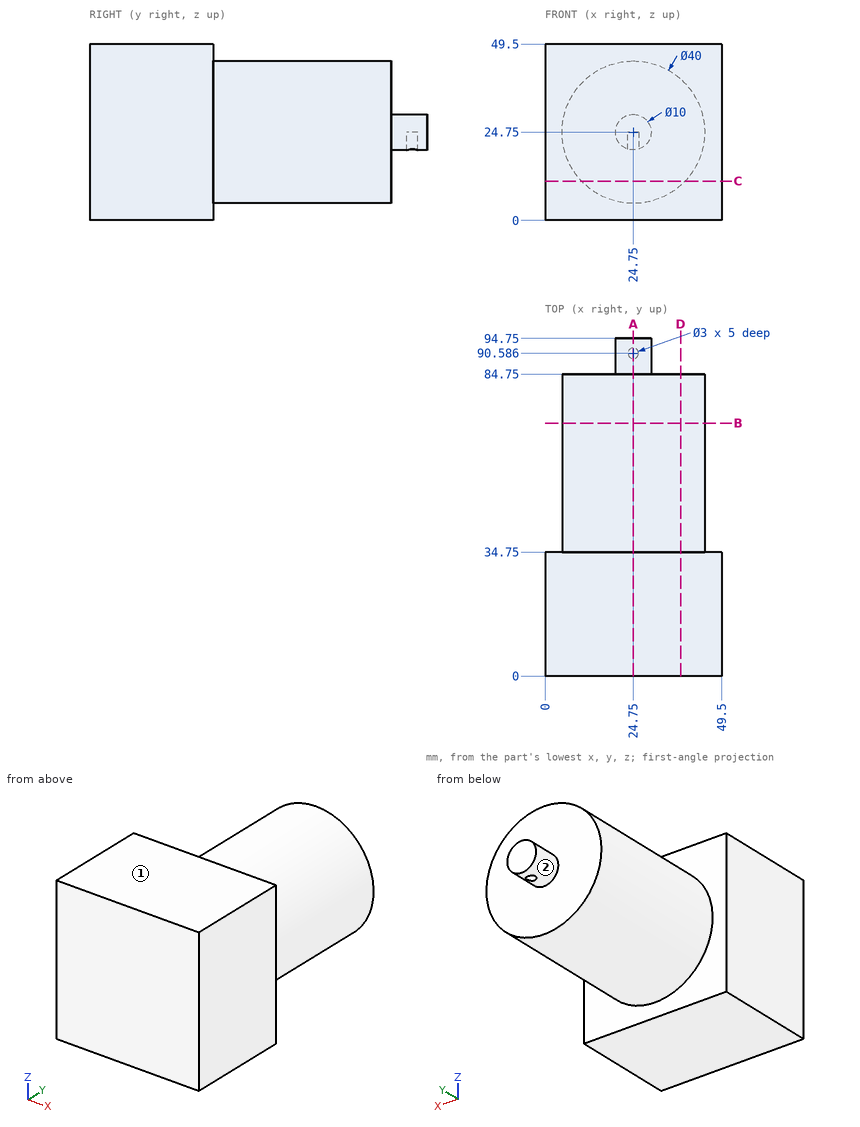
Input: dimensioned drawing with shaded views. Units: mm. Origin: part minimum x, y, z. A direction names the side the tool comes from. Give positions to 0.01 mm unless a question says otherwise; leave off trailing zeros. Write each loop counter-clockwise with the first axis right and the second up, starting at its lowest first coordinate (ties: lowest second). Pieces come first, ordered by that corner, then holes. Notation, with made-up numbers: M 36,88.25 L 65,88.25 A8 ccw 65,102.25 Z; hole C 31,70.25 d11. An arc over 180 degrees is marked long. Return JSON: item names as keys, results as strings. Group by question number.
1) Cut plane B-B, the plane y = 71. Output: boundary loops of the cut face in (x, z).
2) Cut plane A-A, the plane x = 24.75. Output: boundary loops of the cut face in (y, z).
3) Cut plane C-C, the plane z = 11. Output: boundary loops of the cut face in (x, y), plus the area to 3 significant figures.
4) Set-up query: the marked faces 1 and 2. Return all of +Z, -Z, +X, -X, +Y, -Y with unobstructed straight access to the full face (end or side cutting, diameter ignored); none if empty.
5) Material intervals for line 1 along Y through (x, z) = (24.75, 20.8); line 2 along Y through (x, z) = (27, 16.5); line 3 along Y through (x, z) = (6.5, 16), sorted ascending. Write a range as [from, to].
6) Cut plane D-D, the plane x = 38. Output: boundary loops of the cut face in (y, z).
7) Pin query (flat end, axial travel): P1, Ø0.9, axis at x = 24, y = 90.5, coming from the -Z side; P2, Ø3.5, axis at x = 24.75, y = 90.59, coming from the +Z side; P3, Ø2, axis at x = 23, y = 56.5, coming from the -Z side. Return the tip coordinate at first contact, or that it passes through.
Recorded:
{
 "1": {"outline": "C 24.75,24.75 d40"},
 "2": {"outline": "M 0,0 L 34.75,0 L 34.75,4.75 L 84.75,4.75 L 84.75,19.75 L 89.09,19.75 L 89.09,24.75 L 92.09,24.75 L 92.09,19.75 L 94.75,19.75 L 94.75,29.75 L 84.75,29.75 L 84.75,44.75 L 34.75,44.75 L 34.75,49.5 L 0,49.5 Z"},
 "3": {"outline": "M 0,0 L 49.5,0 L 49.5,34.75 L 39.27,34.75 L 39.27,84.75 L 10.23,84.75 L 10.23,34.75 L 0,34.75 Z", "area": "3,170 mm²"},
 "4": {"face 1": "+Z, +X, -X, +Y, -Y", "face 2": "+Y"},
 "5": {"line 1": "y = [0, 89.09], [92.09, 94.75]", "line 2": "y = [0, 84.75]", "line 3": "y = [0, 34.75]"},
 "6": {"outline": "M 0,0 L 34.75,0 L 34.75,9.77 L 84.75,9.77 L 84.75,39.73 L 34.75,39.73 L 34.75,49.5 L 0,49.5 Z"},
 "7": {"P1": "stops at z = 24.75", "P2": "stops at z = 29.75", "P3": "stops at z = 4.76"}
}
